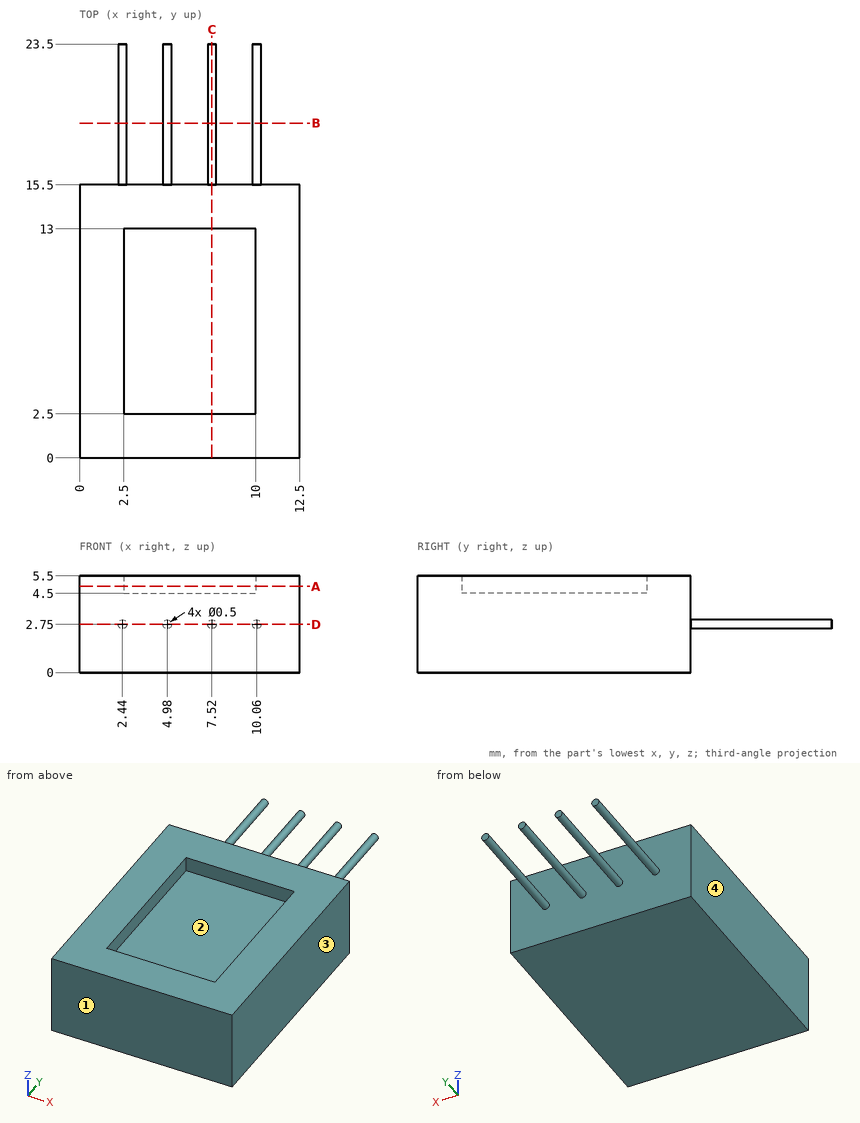
Could you check a few things on this drawing? It's one solid part, dimensions in mm from its lowest x, y, z. Give positions to 0.01 mm unless a question says otherwise; leave off trailing zeros. Order: outer loops, then holes, each group sorted by start corner. A loop starts at its lowest first (then second) coordinate and runs counter-clockwise, first axis right, second up.
1. Suppose I cut it at A-A (z = 4.9). Write out the boundary of the cut face in (x, y), plus the area to 3 significant figures.
Answers below:
outline: (0, 0) - (12.5, 0) - (12.5, 15.5) - (0, 15.5) - close; hole (2.5, 2.5) - (10, 2.5) - (10, 13) - (2.5, 13) - close
area: 115 mm2
2. Suppose I cut it at D-D (z = 2.75). Write out the boundary of the cut face in (x, y).
Answers below:
outline: (0, 0) - (12.5, 0) - (12.5, 15.5) - (10.31, 15.5) - (10.31, 23.5) - (9.81, 23.5) - (9.81, 15.5) - (7.77, 15.5) - (7.77, 23.5) - (7.27, 23.5) - (7.27, 15.5) - (5.23, 15.5) - (5.23, 23.5) - (4.73, 23.5) - (4.73, 15.5) - (2.69, 15.5) - (2.69, 23.5) - (2.19, 23.5) - (2.19, 15.5) - (0, 15.5) - close
3. I need wall thicknesses on L1, parallel to Y at x = 8.25, z = 5; L2, parallel to Y at x = 9, z = 4.15; L3, parallel to X at y = 5, z = 5.05. Which ranges of each line are inside material? Lowest first, please.
Answers below:
L1: y = 0 to 2.5, 13 to 15.5
L2: y = 0 to 15.5
L3: x = 0 to 2.5, 10 to 12.5
4. Suppose I cut it at C-C (x = 7.52). Write out the boundary of the cut face in (y, z).
Answers below:
outline: (0, 0) - (15.5, 0) - (15.5, 2.5) - (23.5, 2.5) - (23.5, 3) - (15.5, 3) - (15.5, 5.5) - (13, 5.5) - (13, 4.5) - (2.5, 4.5) - (2.5, 5.5) - (0, 5.5) - close
5. Suppose I cut it at B-B (y = 19). Write out the boundary of the cut face in (x, z).
Answers below:
outline: circle Ø0.5 at (2.44, 2.75); circle Ø0.5 at (4.98, 2.75); circle Ø0.5 at (7.52, 2.75); circle Ø0.5 at (10.06, 2.75)
6. Thinking about a two-plate mould opening in X: for the marked faces 1, 2, 3 and 4, which applies, +X half, -X half, draft (parallel to the pull), parting line (faces both ways), or undercut?
Answers below:
face 1: draft
face 2: undercut
face 3: +X half
face 4: -X half
7. For pin 1 (0.8 mm diameter, centred on x = 7.5, z = 5, fed in from +Y); pin 2 (4 mm diameter, centred on x = 5.5, y = 9, fed in from +Z), each with a flat end and sliding along its axis, tell me the tip position at first contact or that it passes through.
Answers below:
pin 1: stops at y = 15.5
pin 2: stops at z = 4.5
